Job drawing, mm, ordinate dimensions from the low corner. One solid piece. A direction names the side the tool comes from. Coordinates: 2 decimals unless noted, no trailing zeros. Write each loop counter-clockwise with the first axis right and the second up, starting at its lowest first coordinate (ties: lowest second). Pieces come first, ordered by that corner, then holes.
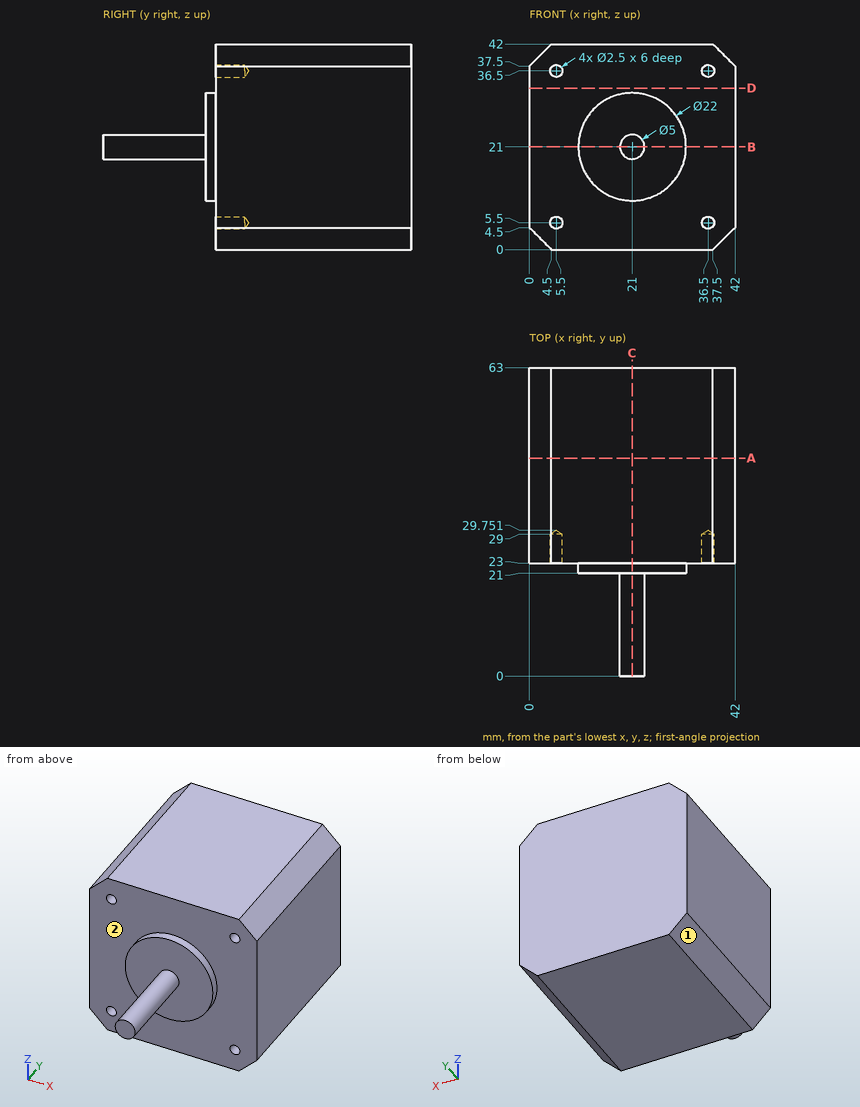
1. Saw through at B-B on z = 21. List the corners of the cut face in (x, y), plus the area to 3 significant figures.
Computed values:
outline: (0, 23) - (10, 23) - (10, 21) - (18.5, 21) - (18.5, 0) - (23.5, 0) - (23.5, 21) - (32, 21) - (32, 23) - (42, 23) - (42, 63) - (0, 63) - close
area: 1,830 mm2
2. 3-axis set-ups, long thin cutter, end or side, ignore diameter. For the marked faces 1 and 2: which of +Z, -Z, +X, -X, +Y, -Y reach the whole face in a straight line?
Computed values:
face 1: -Z, -X, +Y, -Y
face 2: -Y
3. Saw through at C-C on x = 21. List the corners of the cut face in (y, z).
Computed values:
outline: (0, 18.5) - (21, 18.5) - (21, 10) - (23, 10) - (23, 0) - (63, 0) - (63, 42) - (23, 42) - (23, 32) - (21, 32) - (21, 23.5) - (0, 23.5) - close
4. Probe line 1 along X through (y, z) = (26.35, 5.5); line 2 along Y through (x, z) = (6, 34). List the from-to ranges inside material, lowest first.
Computed values:
line 1: x = 0 to 4.25, 6.75 to 35.25, 37.75 to 42
line 2: y = 23 to 63
5. Flat gauge pins, fed straight in: pin 1 (1.5 mm diameter, centred on x = 36.5, z = 36.5, fed in from -Y); pin 2 (2 mm diameter, centred on x = 36.5, z = 5.5, fed in from -Y); pin 3 (3 mm diameter, centred on x = 5.5, z = 5.5, fed in from -Y). Where does each tip first touch, or does it go through?
Computed values:
pin 1: stops at y = 29.3
pin 2: stops at y = 29.15
pin 3: stops at y = 23
6. Saw through at A-A on y = 44.5. List the corners of the cut face in (x, z).
Computed values:
outline: (0, 4.5) - (4.5, 0) - (37.5, 0) - (42, 4.5) - (42, 37.5) - (37.5, 42) - (4.5, 42) - (0, 37.5) - close
7. Saw through at D-D on z = 33. List the corners of the cut face in (x, y), plus the area to 3 significant figures.
Computed values:
outline: (0, 23) - (42, 23) - (42, 63) - (0, 63) - close
area: 1,680 mm2
